Part model, mm, in its own coordinate system. A direction names the side the tool comes from. Round coordinates to 2 decimals unless told otherwise and drop trailing zeros. Loops run counter-clockwise (first coordinate to the right, second up) from the corner with the lowest first, then second, coordinate; pieces in that order, holes last. Notation, with made-up numbers: (60.5, 37) -> (101.5, 37) arc R10 cw to (101.5, 50) -> close; hole circle Ø2 at (67, 76). An arc over 180 degrees is marked (long way). Answer as a JSON object with one key per item and string values. Group by question number.
from build123d import *

# Parameters (mm, degrees)
BOSS_EXTRUDE1_DEPTH = 210.695
FILLET1_R           = 1.651
SKETCH4_R           = 2.585
CUT_EXTRUDE1_DEPTH  = 10
SKETCH9_R           = 3.18
CUT_EXTRUDE2_DEPTH  = 30


with BuildPart() as part:
    # Sketch3 → Boss-Extrude1 (new, symmetric)
    with BuildSketch(Plane.XY):
        Polygon((-25.4, 12.7), (-25.4, -12.7), (25.4, -12.7), (25.4, 12.7), (22.098, 12.7), (22.098, -9.398), (-22.098, -9.398), (-22.098, 12.7), align=None)
    extrude(amount=BOSS_EXTRUDE1_DEPTH, both=True)

    # Fillet1
    fillet1_edges = [part.edges().sort_by_distance(p)[0] for p in [
        (-22.098, -9.398, 0),
        (22.098, -9.398, 0),
    ]]
    fillet(fillet1_edges, radius=FILLET1_R)

    # Sketch4 → Cut-Extrude1 (cut)
    with BuildSketch(Plane(origin=(0, -9.398, 0), x_dir=(1, 0, 0), z_dir=(0, 1, 0))):
        with Locations(Location((-10.530435142, 8.79, 0), (0, 0, 180))):
            Circle(SKETCH4_R)
        with Locations(Location((10.469564858, 8.79, 0), (0, 0, 180))):
            Circle(SKETCH4_R)
        with Locations(Location((-10.530435142, 36.79, 0), (0, 0, 180))):
            Circle(SKETCH4_R)
        with Locations(Location((10.469564858, 36.79, 0), (0, 0, 180))):
            Circle(SKETCH4_R)
        with Locations(Location((-10.530435142, -36.79, 0), (0, 0, 180))):
            Circle(SKETCH4_R)
        with Locations(Location((10.469564858, -36.79, 0), (0, 0, 180))):
            Circle(SKETCH4_R)
        with Locations(Location((10.469564858, -8.79, 0), (0, 0, 180))):
            Circle(SKETCH4_R)
        with Locations(Location((-10.530435142, -8.79, 0), (0, 0, 180))):
            Circle(SKETCH4_R)
    extrude(amount=-CUT_EXTRUDE1_DEPTH, mode=Mode.SUBTRACT)

    # Sketch9 → Cut-Extrude2 (cut, symmetric)
    with BuildSketch(Plane(origin=(0, 0, 0), x_dir=(0, 0, -1), z_dir=(1, 0, 0))):
        with Locations(Location((-62.52, 0, 0), (0, 0, 270))):
            Circle(SKETCH9_R)
        with Locations(Location((62.52, 0, 0), (0, 0, 270))):
            Circle(SKETCH9_R)
    extrude(amount=CUT_EXTRUDE2_DEPTH, both=True, mode=Mode.SUBTRACT)


solid = part.part
Item 1: Band-saw the part on A-A, the plane z = 181.5. List the corners of the cut face in (x, y).
Item 2: Two-plate mould, pull along X, no slides. Class faces 1 (the face through (22.098, 3, 3)), 2 (the face through (2, -10, -210.695)), 3 (the face through (-25.4, 0, 3)): pulls with the +X half, pulls with the -X half, needs draft (parallel to the pull), parting line crosses it, or undercut.
Item 3: Drop a flat-ended pin along its axis: pin 1 Ø6 at (x, z) = (10.47, -8.79) entering from +Y. Give the stop position or say it passes through.
Item 4: Drill centre lines: line 1 (Z direction, x = -24.15, y = 0) (3 decimals); line 2 (X direction, y = -7, z = -77); line 3 (Y direction, x = -24.6, z = 62.52). Where is each one in solid material? Low to high.
Item 5: Which spindle directions (+Z, -Z, +X, -X, +Y, -Y) get a long thin tool onto all of the face, cutting with end or side? Do faces 4 (the face through (0, -9.398, 3)), 5 (the face through (2, -10, 210.695)). Say none if no direction does.
Entries:
{
 "1": {"outline": "(-25.4, -12.7) -> (25.4, -12.7) -> (25.4, 12.7) -> (22.1, 12.7) -> (22.1, -7.75) arc R1.65 cw to (20.45, -9.4) -> (-20.45, -9.4) arc R1.65 cw to (-22.1, -7.75) -> (-22.1, 12.7) -> (-25.4, 12.7) -> close"},
 "2": {"face 1": "undercut", "face 2": "needs draft", "face 3": "pulls with the -X half"},
 "3": {"pin 1": "y = -9.4"},
 "4": {"line 1": "-210.695 to -65.7, -59.34 to 59.34, 65.7 to 210.695", "line 2": "-25.4 to -22.1, 22.1 to 25.4", "line 3": "-12.7 to -3.18, 3.18 to 12.7"},
 "5": {"face 4": "+Z, -Z, +Y", "face 5": "+Z, +X, -X, +Y, -Y"}
}
